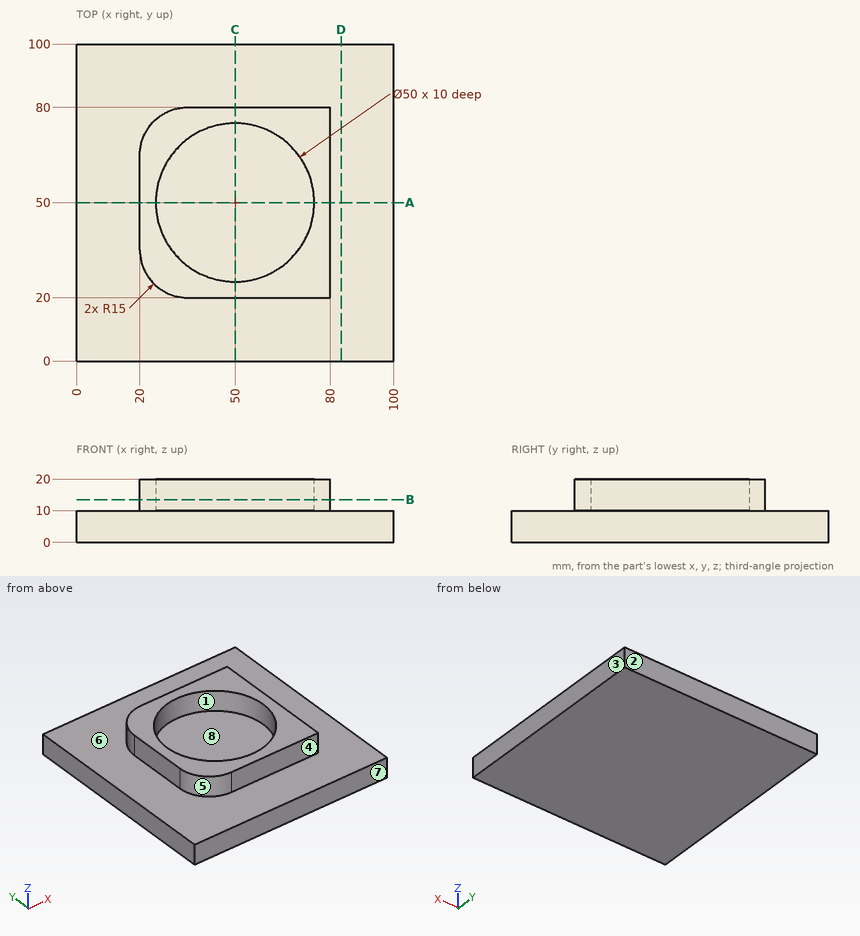
Could you check a few things on this drawing? It's one solid part, dimensions in mm from its lowest x, y, z. A direction names the side the tool comes from. Coordinates: 2 decimals unless noted, no trailing zeros. Write each loop counter-clockwise with the first axis right and the second up, starting at its lowest first coordinate (ties: lowest second). Pieces come first, ordered by that corner, then holes. Notation, with made-up numbers: (52, 83) - (64, 83) arc R24 ccw to (64, 98) - close; hole circle Ø3 at (43.5, 73.5). An arc over 180 degrees is marked (long way). Put each result on its own line as item: value. Start each with the question number.
Q1. I want a section at D-D on x = 83.5. Write out the boundary of the cut face in (y, z).
Q2. Which directions (+Z, -Z, +X, -X, +Y, -Y) give clear straight access to the entire face, cutting with the end or side of a thin tool? Please do the marked faces 1, 2, 3, 4 and 5.
Q3. Please list where these lines run through material, in increasing order: L1, parallel to Y at x = 50, z = 12; L2, parallel to Z at x = 7, y = 48.5; L3, parallel to Y at x = 76, z = 16.25.
Q4. Thinking about a two-plate mould opening in Y: for the marked faces 6, 7 and 8, which applies, pulls with the +Y half, pulls with the -Y half, needs draft (parallel to the pull), parting line crosses it, or undercut?
Q5. I want a section at B-B on z = 13.5. Write out the boundary of the cut face in (x, y).
Q6. I'm going to push flat-ended pins straight in: P1, Ø11, axis at x = 47, z = 17, coming from the +Y side; P2, Ø3, axis at x = 50.5, z = 14, coming from the -Y side; P3, Ø10, axis at x = 12.5, z = 6.5, coming from the -Y side; P4, Ø3, axis at x = 44, y = 61.5, coming from the +Z side. Where does each tip first touch, or does it pass through?
Q7. I want a section at A-A on y = 50. Write out the boundary of the cut face in (x, z).
Checks:
1. outline: (0, 0) - (100, 0) - (100, 10) - (0, 10) - close
2. face 1: +Z
2. face 2: +Z, -Z, +X, -X, +Y
2. face 3: +Z, -Z, +X, +Y, -Y
2. face 4: +Z, +X, -X, -Y
2. face 5: +Z, -X, -Y
3. L1: 20 to 25, 75 to 80
3. L2: 0 to 10
3. L3: 20 to 80
4. face 6: needs draft
4. face 7: pulls with the -Y half
4. face 8: undercut
5. outline: (20, 35) arc R15 ccw to (35, 20) - (80, 20) - (80, 80) - (35, 80) arc R15 ccw to (20, 65) - close; hole circle Ø50 at (50, 50)
6. P1: y = 80
6. P2: y = 20
6. P3: y = 0
6. P4: z = 10
7. outline: (0, 0) - (100, 0) - (100, 10) - (80, 10) - (80, 20) - (75, 20) - (75, 10) - (25, 10) - (25, 20) - (20, 20) - (20, 10) - (0, 10) - close
